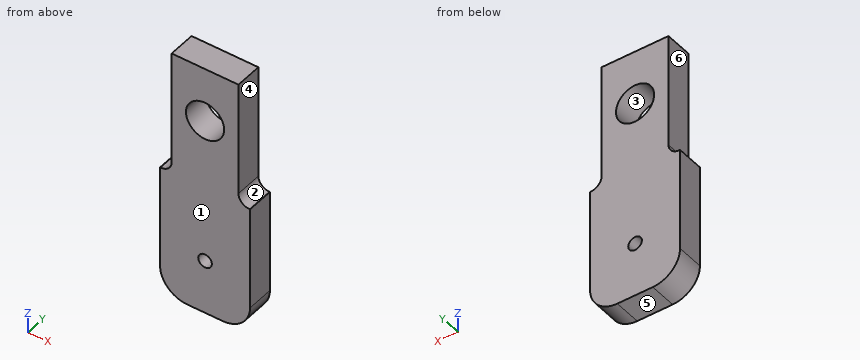
Autodesk Inventor part; units mm, degrees
ref_plane "YZ Plane" through (0, 0, 0) normal (1, 0, 0) x (0, 1, 0)
ref_plane "XZ Plane" through (0, 0, 0) normal (0, 1, 0) x (-1, 0, 0)
ref_plane "XY Plane" through (0, 0, 0) normal (0, 0, 1) x (1, 0, 0)
sketch "Sketch1" plane through (0, 0, 0) normal (0, 1, 0) x (-1, 0, 0)
  line L0 (15.5575, -24.13) -> (15.5575, 29.21)
  line L1 (15.5575, 29.21) -> (-15.5575, 29.21)
  line L2 (-15.5575, 29.21) -> (-15.5575, -24.13)
  line L3 (-15.5575, -29.21) -> (15.5575, 29.21) construction
  line L4 (15.5575, -29.21) -> (-15.5575, 29.21) construction
  line L5 (20.6375, -29.21) -> (20.955, -29.21)
  line L6 (20.955, -29.21) -> (20.955, -77.47)
  line L7 (8.255, -90.17) -> (-8.255, -90.17)
  line L8 (-20.955, -77.47) -> (-20.955, -29.21)
  line L9 (-20.955, -29.21) -> (-20.6375, -29.21)
  arc A0 (15.5575, -24.13) -> (20.6375, -29.21) centre (20.6375, -24.13) ccw
  arc A1 (-20.6375, -29.21) -> (-15.5575, -24.13) centre (-20.6375, -24.13) ccw
  circle A2 centre (0, 3.81) radius 8.89
  arc A3 (8.255, -90.17) -> (20.955, -77.47) centre (8.255, -77.47) ccw
  arc A4 (-20.955, -77.47) -> (-8.255, -90.17) centre (-8.255, -77.47) ccw
  point P0 (0, 0)
  point P1 (20.955, -90.17)
  point P2 (-20.955, -90.17)
  dimension "d0" = 5.08
  dimension "d1" = 31.115
  dimension "d2" = 41.91
  dimension "d3" = 60.96
  dimension "d4" = 119.38
  dimension "d5" = 17.78
  dimension "d6" = 25.4
  dimension "d7" = 12.7
extrude "Extrusion1" add sketch "Sketch1" along normal blind 12.7
sketch "Sketch2" plane through (0, 12.7, 0) normal (0, 1, 0) x (1, 0, 0)
  line L0 (-8.255, 90.17) -> (8.255, 90.17)
  point P0 (0, 0)
  point P1 (0, 64.77)
  dimension "d19" = 25.4
hole "Hole2" at (0, 12.7, -64.77) direction (0, -1, 0) diameter 6.35 end through all
properties part number "Fixture_Airpot_Support"
Model file for the job. Use its own axes, mm. Face numbers are marked on the shaded views. A direction names the side the tool comes from. Coordinates: 2 decimals unless noted, no trailing zeros. Write each loop counter-clockwise with the first axis right and the second up, starting at its lowest first coordinate (ties: lowest second). Pieces come first, ordered by that corner, then holes. Notation, with made-up numbers: (-36, 87) - (-5, 87) arc R13 cw to (-5, 112) - close; hole circle Ø7 at (-29, -3.75). An arc over 180 degrees is marked (long way). Use a Markdown table: item, result. Add a question column.
Item 1: Band-saw the part on C-C, the plane z = -64.77. Write the cut outline in (x, y) (3 decimals).
Item 2: Two-plate mould, pull along X, no slides. Class the marked faces 1, 2 and 3: pulls with the +X half, pulls with the -X half, needs draft (parallel to the pull), parting line crosses it, or undercut.
Item 3: 3-axis set-ups, long thin cutter, end or side, ignore diameter. For the marked faces 4, 5 and 6: which of +Z, -Z, +X, -X, +Y, -Y reach the whole face in a straight line?
Item 4: Band-saw the part on D-D, the plane z = -17. Write the cut outline in (x, y).
Item 5: Band-saw the part on B-B, the plane y = 2. Give the number of separate pieces and of enclosed holes in the cut face, and give its area (3 significant figures).
Item 6: Drop flat-ended pins along their axis: pin 1 (16 mm diameter, centred on x = 0, z = 3.81, fed in from -Y); pin 2 (1.5 mm diameter, centred on y = 3.5, z = 7, fed in from -X); pin 3 (3 mm diameter, centred on y = 3.5, z = -26, fed in from -X); pin 4 (4 mm diameter, centred on y = 8.5, z = 5.5, fed in from +X). Give the stop position or say it passes through.
Item 7: Drill centre lines: line 1 along Z through (x, y) = (0, 5.5) (3 decimals); line 2 along X through (y, z) = (1, 21.5); line 3 along X through (y, z) = (9.5, -64.77) (3 decimals). Where is each one in solid material? Low to high.
Item 8: Band-saw the part on A-A, the plane z = 3.81. Write the cut outline in (x, y), and give its area (3 significant figures).
A:
| question | item | result |
|---|---|---|
| 1 | outline | (-20.955, 0) - (-3.175, 0) - (-3.175, 12.7) - (-20.955, 12.7) - close; (3.175, 0) - (20.955, 0) - (20.955, 12.7) - (3.175, 12.7) - close |
| 2 | face 1 | needs draft |
| 2 | face 2 | pulls with the +X half |
| 2 | face 3 | undercut |
| 3 | face 4 | +Z, +X, +Y, -Y |
| 3 | face 5 | -Z, +X, -X, +Y, -Y |
| 3 | face 6 | +Z, -X, +Y, -Y |
| 4 | outline | (-15.56, 0) - (15.56, 0) - (15.56, 12.7) - (-15.56, 12.7) - close |
| 5 | separate pieces | 1 |
| 5 | enclosed holes | 2 |
| 5 | area | 4,030 mm² |
| 6 | pin 1 | passes through |
| 6 | pin 2 | stops at x = -15.56 |
| 6 | pin 3 | stops at x = -16.84 |
| 6 | pin 4 | stops at x = 15.56 |
| 7 | line 1 | z = -90.17 to -67.945, -61.595 to -5.08, 12.7 to 29.21 |
| 7 | line 2 | x = -15.56 to 15.56 |
| 7 | line 3 | x = -20.955 to -3.175, 3.175 to 20.955 |
| 8 | outline | (-15.56, 0) - (-8.89, 0) - (-8.89, 12.7) - (-15.56, 12.7) - close; (8.89, 0) - (15.56, 0) - (15.56, 12.7) - (8.89, 12.7) - close |
| 8 | area | 169 mm² |
